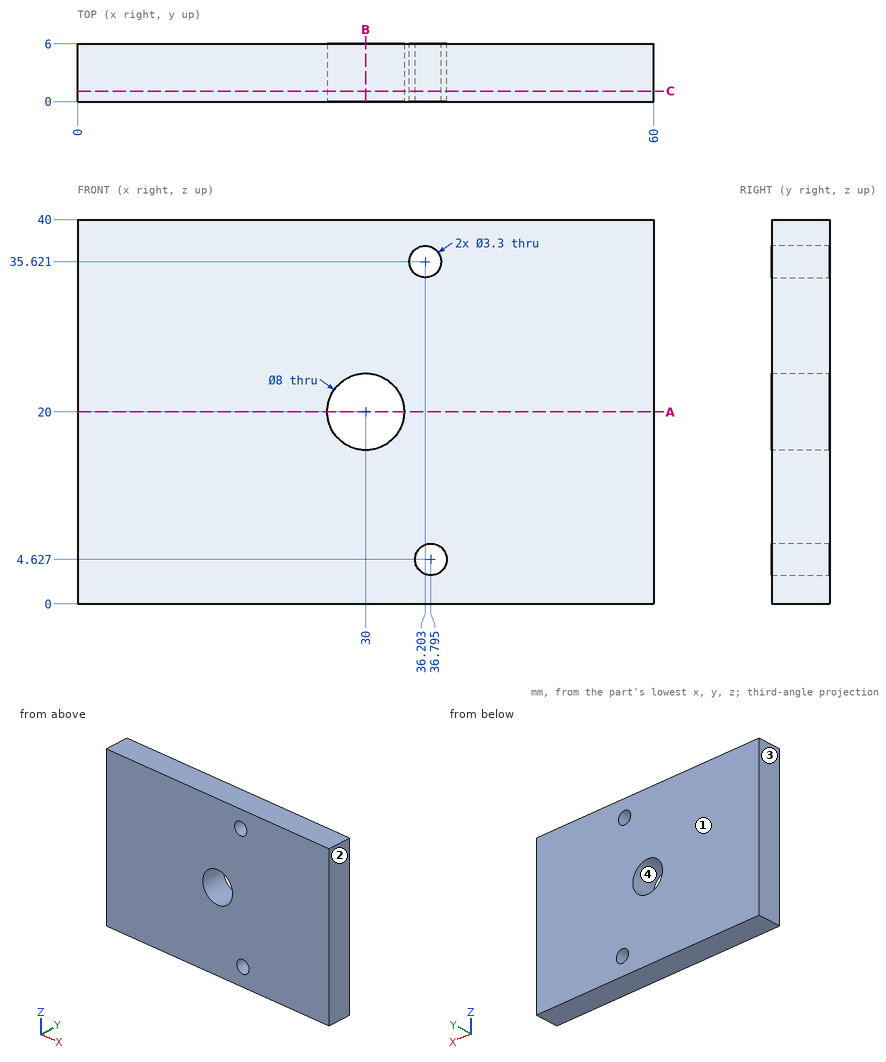
For this review, use the dimensioned drawing (mm, ordinates from the lowest corner) and the shaded views. Coordinates: 2 decimals unless noted, no trailing zeros. Order: outer loops, then holes, each group sorted by start corner. A loop starts at its lowest first (then second) coordinate and runs counter-clockwise, first axis right, second up. Notation, with made-up numbers: M -10.75,-38 L 12.25,-38 A28 ccw 12.25,-9 Z; hole C 54.25,-1 d7. An arc over 180 degrees is marked long. Answer as a JSON object with one key per item and string values. Group by question number.
1) For pin 1 (5 mm diameter, centred on x = 30, z = 20, fed in from -Y), flat-tipped, find the tip position at first contact; note if it passes through.
2) Add section C-C, the plane y = 1.1. Count the separate pieces of the cut face and the enclosed holes in it, then the cut area to 3 significant figures.
3) Add section B-B, the plane x = 30. Write out the cut boundary in (y, z).
4) Add section A-A, the plane z = 20. Write out the cut boundary in (x, y).
5) Mouldability with a two-part tool opening along X and no side actions: class the marked faces 1, 2, 3 and 4 as pulls with the +X half, pulls with the -X half, needs draft (parallel to the pull), parting line crosses it, or undercut.
6) Wall thickness on L1, parallel to Z at x = 37, y = 4.5 (1 decimal); L2, parallel to X at y = 1.35, z = 20; L3, parallel to X at y = 1.3, z = 23 (1 decimal): over which ranges is each line inside the solid? List them lowest first.
Computed values:
{
 "1": {"pin 1": "passes through"},
 "2": {"separate pieces": "1", "enclosed holes": "3", "area": "2,330 mm^2"},
 "3": {"outline": "M 0,0 L 6,0 L 6,16 L 0,16 Z; M 0,24 L 6,24 L 6,40 L 0,40 Z"},
 "4": {"outline": "M 0,0 L 26,0 L 26,6 L 0,6 Z; M 34,0 L 60,0 L 60,6 L 34,6 Z"},
 "5": {"face 1": "needs draft", "face 2": "pulls with the +X half", "face 3": "pulls with the -X half", "face 4": "undercut"},
 "6": {"L1": "z = 0 to 3, 6.3 to 34.2, 37.1 to 40", "L2": "x = 0 to 26, 34 to 60", "L3": "x = 0 to 27.4, 32.6 to 60"}
}
